Check sheet for the modelled part. Datum: model origin and axes. Units: mm. A direction names the side the tool comes from. Coordinates: 2 decimals unless noted, no trailing zeros. Loops run counter-clockwise (first coordinate to the right, second up) from the corner with the lowest first, then second, coordinate; pieces in that order, holes last. Notation, with made-up numbers: (80, -2) -> (103, -2) arc R31 ccw to (103, 29) -> close; hole circle Ø5 at (14.25, -6.5). An arc over 180 degrees is marked (long way). Use one line per item in the form item = value.
from build123d import *

# Parameters (mm, degrees)
SALIENTE_EXTRUIR1_DEPTH = 3
REDONDEO1_R             = 2


with BuildPart() as part:
    # Croquis1 → Saliente-Extruir1 (new body)
    with BuildSketch(Plane(origin=(0, 0, 0), x_dir=(1, 0, 0), z_dir=(0, 1, 0))):
        Polygon((0, 0), (2.5, 0), (2.5, 3), (5.5, 3), (5.5, 0), (106.1, 0), (106.1, 3), (109.1, 3), (109.1, 0), (111.1, 0), (111.1, 5), (0, 5), align=None)
    extrude(amount=SALIENTE_EXTRUIR1_DEPTH)

    # Redondeo1
    redondeo1_edges = [part.edges().sort_by_distance(p)[0] for p in [
        (0, 1.5, -5),
        (111.1, 1.5, -5),
    ]]
    fillet(redondeo1_edges, radius=REDONDEO1_R)


solid = part.part
(1) Scan lines: line 1 along X through (y, z) = (1.8, -1.6); line 2 along X through (y, z) = (2.3, -3.1); line 3 along X through (y, z) = (0.85, -4.65). Record each from-to range of solid material in increasing order.
Established:
line_1 = 0 to 2.5, 5.5 to 106.1, 109.1 to 111.1
line_2 = 0 to 111.1
line_3 = 0.87 to 110.23
(2) Mould release check, pull along X, two halves, no side actions. Record for faces 1 (the flat face through (55, 0, -3)), 2 (the flat face through (0, 1, -2)), 3 (the flat face through (4, 1, -3)), 4 (the flat face through (111.1, 1, -1)): +X half, -X half, draft (parallel to the pull), parting line (faces both ways), or undercut.
Established:
face_1 = draft
face_2 = -X half
face_3 = undercut
face_4 = +X half
(3) Section check A-A, the plane z = -1.35. Record the boundary of the cut face in (x, y), plus the area to 3 significant figures.
Established:
outline = (0, 0) -> (2.5, 0) -> (2.5, 3) -> (0, 3) -> close; (5.5, 0) -> (106.1, 0) -> (106.1, 3) -> (5.5, 3) -> close; (109.1, 0) -> (111.1, 0) -> (111.1, 3) -> (109.1, 3) -> close
area = 315 mm²
(4) Tool access check on faces 5 (the flat face through (5.5, 1, -2)), 6 (the cylindrical face through (110.53, 1.52, -4.4)). Record the directions out of +Z, -Z, +X, -X, +Y, -Y that give a thin tool (end or side, any length) a straight path to the whole face; none if there is none.
Established:
face_5 = +Z, +Y, -Y
face_6 = -Z, +X, +Y, -Y
(5) Go/stop test with a flat-tipped pin: P1, Ø1.5, axis at x = 38.5, z = -1.5, coming from the -Y side. Record where the tip stops, or that it passes through.
Established:
P1 = 0
(6) Section check B-B, the plane y = 1.6. Record the boundary of the cut face in (x, z).
Established:
outline = (0, -3) arc R2 ccw to (2, -5) -> (109.1, -5) arc R2 ccw to (111.1, -3) -> (111.1, 0) -> (109.1, 0) -> (109.1, -3) -> (106.1, -3) -> (106.1, 0) -> (5.5, 0) -> (5.5, -3) -> (2.5, -3) -> (2.5, 0) -> (0, 0) -> close
